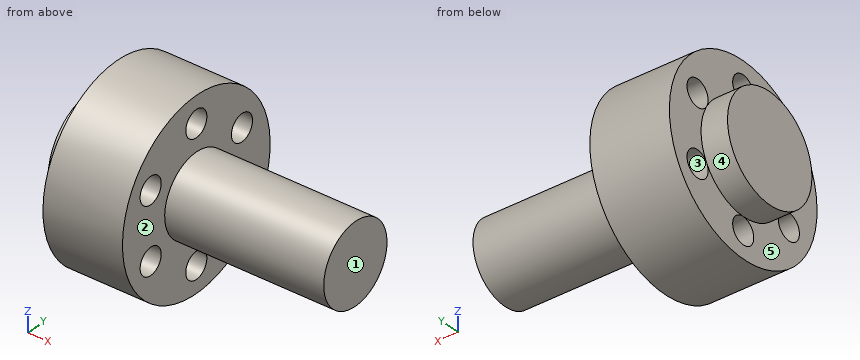
```python
from build123d import *

# Parameters (mm, degrees)
SKETCH_2_R          = 5
CUT_EXTRUDE_1_DEPTH = 112.579568022
SKETCH_3_R          = 5
CUT_EXTRUDE_2_DEPTH = 112.579568022
SKETCH_4_R          = 5
CUT_EXTRUDE_3_DEPTH = 112.579568022
SKETCH_5_R          = 5
CUT_EXTRUDE_4_DEPTH = 112.579568022
SKETCH_6_R          = 5
CUT_EXTRUDE_5_DEPTH = 112.579568022
SKETCH_7_R          = 5
CUT_EXTRUDE_6_DEPTH = 112.579568022


with BuildPart() as part:
    # Эскиз1 → Повернуть1 (revolve)
    with BuildSketch(Plane.XY, mode=Mode.PRIVATE) as revolve_1_sk:
        Polygon((0, 0), (100, 0), (100, 15), (40, 15), (40, 35), (10, 35), (10, 20), (0, 20), align=None)
    revolve(revolve_1_sk.sketch.rotate(Axis((0, 0, 0), (1, 0, 0)), 90), axis=Axis((0, 0, 0), (1, 0, 0)))

    # Эскиз2 → Вырез-Вытянуть1 (cut, through all)
    with BuildSketch(Plane(origin=(0, 0, 0), x_dir=(0, 0, -1), z_dir=(1, 0, 0))):
        with Locations(Location((25, 0, 0), (0, 0, 180))):
            Circle(SKETCH_2_R)
    extrude(amount=CUT_EXTRUDE_1_DEPTH, mode=Mode.SUBTRACT)

    # Эскиз3 → Вырез-Вытянуть2 (cut, through all)
    with BuildSketch(Plane(origin=(0, 0, 0), x_dir=(0, 0, -1), z_dir=(1, 0, 0))):
        with Locations(Location((12.5, 21.650635095, 0), (0, 0, 180))):
            Circle(SKETCH_3_R)
    extrude(amount=CUT_EXTRUDE_2_DEPTH, mode=Mode.SUBTRACT)

    # Эскиз4 → Вырез-Вытянуть3 (cut, through all)
    with BuildSketch(Plane(origin=(0, 0, 0), x_dir=(0, 0, -1), z_dir=(1, 0, 0))):
        with Locations(Location((-12.5, 21.650635095, 0), (0, 0, 180))):
            Circle(SKETCH_4_R)
    extrude(amount=CUT_EXTRUDE_3_DEPTH, mode=Mode.SUBTRACT)

    # Эскиз5 → Вырез-Вытянуть4 (cut, through all)
    with BuildSketch(Plane(origin=(0, 0, 0), x_dir=(0, 0, -1), z_dir=(1, 0, 0))):
        with Locations(Location((-25, 0, 0), (0, 0, 180))):
            Circle(SKETCH_5_R)
    extrude(amount=CUT_EXTRUDE_4_DEPTH, mode=Mode.SUBTRACT)

    # Эскиз6 → Вырез-Вытянуть5 (cut, through all)
    with BuildSketch(Plane(origin=(0, 0, 0), x_dir=(0, 0, -1), z_dir=(1, 0, 0))):
        with Locations(Location((-12.5, -21.650635095, 0), (0, 0, 180))):
            Circle(SKETCH_6_R)
    extrude(amount=CUT_EXTRUDE_5_DEPTH, mode=Mode.SUBTRACT)

    # Эскиз7 → Вырез-Вытянуть6 (cut, through all)
    with BuildSketch(Plane(origin=(0, 0, 0), x_dir=(0, 0, -1), z_dir=(1, 0, 0))):
        with Locations(Location((12.5, -21.650635095, 0), (0, 0, 180))):
            Circle(SKETCH_7_R)
    extrude(amount=CUT_EXTRUDE_6_DEPTH, mode=Mode.SUBTRACT)


solid = part.part
```
Read the model definition and answer for the solid it produces. Units are mm, in the model's axes. Face numbers are marked on the shaded views. A direction names the side the tool comes from. Coordinates: 2 decimals unless noted, no trailing zeros. Order: outer loops, then holes, each group sorted by start corner. A loop starts at its lowest first (then second) coordinate and runs counter-clockwise, first axis right, second up. Notation, with made-up numbers: (-29, 3) - (13, 3) arc R27 cw to (13, 36) - close; hole circle Ø1 at (69, -15). An arc over 180 degrees is marked (long way). Answer as a JSON object with one key per item and string values. Group by question number.
Item 1: Section C-C (y = 2) is taken. Give the vertices of the cut face in (x, z), plus the area to 3 significant figures.
Item 2: Section A-A (z = 0) is taken. Give the vertices of the cut face in (x, y).
Item 3: Section D-D (z = 12.5) is taken. Give the vertices of the cut face in (x, y), plus the area to 3 significant figures.
Item 4: A tool of negligible diameter and unlimited length cuts with its end or side. For the marked faces 1 and 2, from which of +Z, -Z, +X, -X, +Y, -Y can it reach the whole face along a straight path? Write none if from no direction.
Item 5: Flat-ended cylindrical pins translate along their axes: P1, Ø16, axis at y = 0, z = -25, coming from the +X side; P2, Ø1.5, axis at x = 28.5, y = 19.5, coming from the -Z side; P3, Ø6, axis at x = 11, y = -22.5, coming from the +Z side. Find the tip coordinate at first contact, or state that the pin passes through.
Item 6: Section B-B (z = -25) is taken. Give the vertices of the cut face in (x, y).
Item 7: The mould has two halves that part along Z. Classify the marked faces 3, 4 and 5: +Z half, -Z half, draft (parallel to the pull), parting line (faces both ways), or undercut.
Item 8: Consider probe 1 along Y at (x, z) = (32.75, 12.5); probe 2 along Z at (x, y) = (16.5, 20); probe 3 along Y at (x, z) = (33.5, -11.5). Determine where each line is inside the solid, lowest interval first. Write a range as from..to.
Results are:
{
 "1": {"outline": "(0, -19.9) - (10, -19.9) - (10, -20.42) - (40, -20.42) - (40, -14.87) - (100, -14.87) - (100, 14.87) - (40, 14.87) - (40, 20.42) - (10, 20.42) - (10, 19.9) - (0, 19.9) - close; (10, -34.94) - (40, -34.94) - (40, -29.58) - (10, -29.58) - close; (10, 29.58) - (40, 29.58) - (40, 34.94) - (10, 34.94) - close", "area": "3,730 mm^2"},
 "2": {"outline": "(0, -20) - (10, -20) - (10, -35) - (40, -35) - (40, -15) - (100, -15) - (100, 15) - (40, 15) - (40, 35) - (10, 35) - (10, 20) - (0, 20) - close"},
 "3": {"outline": "(0, -15.61) - (10, -15.61) - (10, -16.65) - (40, -16.65) - (40, -8.29) - (100, -8.29) - (100, 8.29) - (40, 8.29) - (40, 16.65) - (10, 16.65) - (10, 15.61) - (0, 15.61) - close; (10, -32.69) - (40, -32.69) - (40, -26.65) - (10, -26.65) - close; (10, 26.65) - (40, 26.65) - (40, 32.69) - (10, 32.69) - close", "area": "2,670 mm^2"},
 "4": {"face 1": "+Z, -Z, +X, +Y, -Y", "face 2": "+X"},
 "5": {"P1": "stops at x = 40", "P2": "stops at z = -29.55", "P3": "stops at z = 29.06"},
 "6": {"outline": "(10, -24.49) - (40, -24.49) - (40, -5) - (10, -5) - close; (10, 5) - (40, 5) - (40, 24.49) - (10, 24.49) - close"},
 "7": {"face 3": "undercut", "face 4": "parting line", "face 5": "draft"},
 "8": {"probe 1": "y = -32.69..-26.65, -16.65..16.65, 26.65..32.69", "probe 2": "z = -28.72..-17.22, -7.78..7.78, 17.22..28.72", "probe 3": "y = -33.06..-26.55, -16.75..16.75, 26.55..33.06"}
}
